Verification items for the finished model (mm, model axes). Coordinates: 2 decimals unless noted, no trailing zeros. Write each loop counter-clockwise with the first axis right and the second up, starting at its lowest first coordinate (ties: lowest second). Pieces come first, ordered by that corner, then holes. Notation, with made-up numbers: (10.5, 47) -> (69.5, 47) arc R20 ccw to (69.5, 84) -> close; hole circle Ø8 at (39.5, 86). An arc over 180 degrees is marked (long way). Answer in a Markdown table with one row per item.
Autodesk Inventor part; units mm, degrees
ref_plane "YZ Plane" through (0, 0, 0) normal (1, 0, 0) x (0, 1, 0)
ref_plane "XZ Plane" through (0, 0, 0) normal (0, 1, 0) x (-1, 0, 0)
ref_plane "XY Plane" through (0, 0, 0) normal (0, 0, 1) x (1, 0, 0)
sketch "Sketch1" plane through (0, 0, 0) normal (0, 0, 1) x (1, 0, 0)
  circle A0 centre (0, 0) radius 12.5
  circle A1 centre (0, 0) radius 27.5
  dimension "d2" = 25
  dimension "d3" = 55
extrude "Extrusion1" add sketch "Sketch1" along normal blind 1
sketch "Sketch2" plane through (0, 0, 1) normal (0, 0, 1) x (1, 0, 0)
  circle A0 centre (0, 0) radius 23.75 construction
  point P0 (23.75, 0)
  dimension "d4" = 47.5
hole "Hole1" at (23.75, 0, 1) direction (0, 0, -1) diameter 3.4 end through all
pattern_circular "Circular Pattern1" count 4 over 360 about axis through (0, 0, 0) along (0, 0, 1) of "Hole1"
sketch "Sketch3" plane through (0, 0, 1) normal (0, 0, 1) x (1, 0, 0)
  line L0 (-30, 30) -> (30, 30)
  line L1 (30, 30) -> (30, 20)
  line L2 (30, 20) -> (-30, 20)
  line L3 (-30, 20) -> (-30, 30)
  point P0 (0, 0)
  point P1 (0, 20)
  dimension "d15" = 20
  dimension "d16" = 60
  dimension "d17" = 10
extrude "Extrusion2" cut sketch "Sketch3" against normal through all
mirror "Mirror1" about plane through (0, 0, 0) normal (0, 1, 0) of "Extrusion2"
fillet "Fillet2" radius 2 4 edges at (-18.8746, 20, 0.5) (18.8746, 20, 0.5) (-18.8746, -20, 0.5) (18.8746, -20, 0.5)
properties part number "Plasma Box Slit" material "Stainless Steel"
1. Thickness scan on line 1 (X direction, y = 1.5, z = 0.9); line 2 (Y direction, x = 0, z = 0.45); line 3 (X direction, y = -1, z = 0.75). Record the ranges inside material, lowest first. Write a range as from..to.
Geometry says:
| item | result |
|---|---|
| line 1 | -27.46..-24.55, -22.95..-12.41, 12.41..22.95, 24.55..27.46 |
| line 2 | -20..-12.5, 12.5..20 |
| line 3 | -27.48..-25.12, -22.38..-12.46, 12.46..22.38, 25.12..27.48 |
2. Section check B-B, the plane z = 0.3. Record the boundary of the cut face in (x, y).
Geometry says:
| item | result |
|---|---|
| outline | (-19.48, -19.41) arc R2 ccw to (-18.06, -20) -> (18.06, -20) arc R2 ccw to (19.48, -19.41) arc R27.5 ccw to (19.48, 19.41) arc R2 ccw to (18.06, 20) -> (-18.06, 20) arc R2 ccw to (-19.48, 19.41) arc R27.5 ccw to start; hole circle Ø3.4 at (-23.75, 0); hole circle Ø25 at (0, 0); hole circle Ø3.4 at (23.75, 0) |
3. Section check D-D, the plane y = -7. Record the boundary of the cut face in (x, z), plus the area to 3 significant figures.
Geometry says:
| item | result |
|---|---|
| outline | (-26.59, 0) -> (-10.36, 0) -> (-10.36, 1) -> (-26.59, 1) -> close; (10.36, 0) -> (26.59, 0) -> (26.59, 1) -> (10.36, 1) -> close |
| area | 32.5 mm^2 |
4. Section check A-A, the plane y = 0. Record the boundary of the cut face in (x, z).
Geometry says:
| item | result |
|---|---|
| outline | (-27.5, 0) -> (-25.45, 0) -> (-25.45, 1) -> (-27.5, 1) -> close; (-22.05, 0) -> (-12.5, 0) -> (-12.5, 1) -> (-22.05, 1) -> close; (12.5, 0) -> (22.05, 0) -> (22.05, 1) -> (12.5, 1) -> close; (25.45, 0) -> (27.5, 0) -> (27.5, 1) -> (25.45, 1) -> close |
5. Depth check by flat-ended pin: P1, Ø4, axis at x = 23.75, y = 0, coming from the +Z side. Enter the tip coordinate at first touch or a pass-through.
Geometry says:
| item | result |
|---|---|
| P1 | z = 1 |
6. Section check C-C, the plane x = 0. Record the boundary of the cut face in (y, z), plus the area to 3 significant figures.
Geometry says:
| item | result |
|---|---|
| outline | (-20, 0) -> (-12.5, 0) -> (-12.5, 1) -> (-20, 1) -> close; (12.5, 0) -> (20, 0) -> (20, 1) -> (12.5, 1) -> close |
| area | 15.0 mm^2 |
7. Mould release check, pull along X, two halves, no side actions. Record for faces 1 (the cylindrical face through (-27.5, -0.3, 0.5)), 2 (the flat face through (-13, 0, 1)), 3 (the cylindrical face through (22.064, 0.221, 0.493)), 4 (the cylindrical face through (-22.064, -0.221, 0.493)): released by +X, released by -X, zero draft, split by the parting line, or undercut.
Geometry says:
| item | result |
|---|---|
| face 1 | released by -X |
| face 2 | zero draft |
| face 3 | undercut |
| face 4 | undercut |
